Verification items for this drawing (mm, ordinates from the low corner). Round coordinates to 2 decimals unless told otherwise and drop trailing zeros. Write each loop counter-clockwise with the first axis right and the second up, starting at its lowest first coordinate (ties: lowest second). Pieces come first, ordered by that corner, then holes.
Item 1: Scan lines: probe 1 along Y at (x, z) = (74.5, 0.35); probe 2 along X at (y, z) = (25, 0.2). Record each from-to range of solid material in increasing order.
Item 2: Cross-section at A-A (x = 74.5). Enter the section's corners in (y, z).
Item 3: Cross-section at B-B (y = 3). Enter the section's corners in (x, z), then the cut area to 3 significant figures.
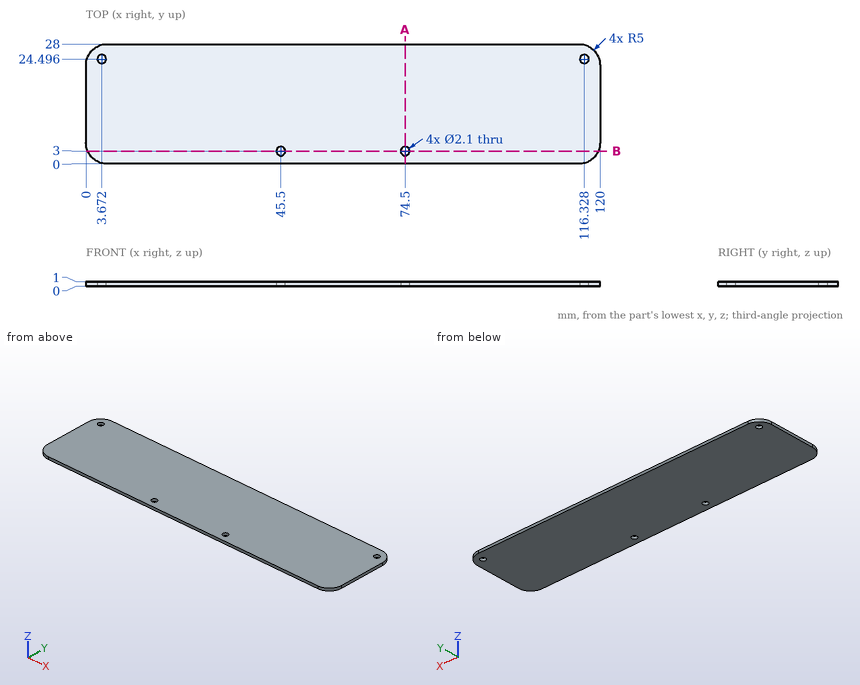
Resolved:
1. probe 1: y = 0 to 1.95, 4.05 to 28
1. probe 2: x = 0.42 to 2.75, 4.59 to 115.41, 117.25 to 119.58
2. outline: (0, 0) - (1.95, 0) - (1.95, 1) - (0, 1) - close; (4.05, 0) - (28, 0) - (28, 1) - (4.05, 1) - close
3. outline: (0.42, 0) - (44.45, 0) - (44.45, 1) - (0.42, 1) - close; (46.55, 0) - (73.45, 0) - (73.45, 1) - (46.55, 1) - close; (75.55, 0) - (119.58, 0) - (119.58, 1) - (75.55, 1) - close
3. area: 115 mm2
